Source: CAD feature listing. Evaluate the final solid. Frame: model axes, mm. Face numbers are marked on the shaded views. A direction names the side the tool comes from. Coordinates: 2 decimals unless noted, no trailing zeros. Loops run counter-clockwise (first coordinate to the right, second up) from the corner with the lowest first, then second, coordinate; pieces in that order, holes last. Notation, with made-up numbers: (47.25, 89) - (90.25, 89) arc R8 cw to (90.25, 102) - close; hole circle Ø1 at (70, 57.5). An arc over 180 degrees is marked (long way). Use one line per item in the form item = value. Start each with the question number.
from build123d import *

# Parameters (mm, degrees)
SKETCH1_W           = 36
SKETCH1_H           = 35
BOSS_EXTRUDE1_DEPTH = 11
SKETCH1_3_W         = 15
SKETCH1_3_H         = 35
BOSS_EXTRUDE2_DEPTH = 15.2
SKETCH2_W           = 31
SKETCH2_H           = 11.2
CUT_EXTRUDE1_DEPTH  = 1


with BuildPart() as part:
    # Sketch1 → Boss-Extrude1 (new body)
    with BuildSketch(Plane(origin=(0, 0, 0), x_dir=(1, 0, 0), z_dir=(0, 1, 0))):
        with Locations((-7.5, 0)):
            Rectangle(SKETCH1_W, SKETCH1_H)
    extrude(amount=BOSS_EXTRUDE1_DEPTH)

    # Sketch1<3> → Boss-Extrude2 (add)
    with BuildSketch(Plane(origin=(0, 0, 0), x_dir=(1, 0, 0), z_dir=(0, 1, 0))):
        with Locations((18, 0)):
            Rectangle(SKETCH1_3_W, SKETCH1_3_H)
    extrude(amount=BOSS_EXTRUDE2_DEPTH)

    # Sketch2 → Cut-Extrude1 (cut)
    with BuildSketch(Plane(origin=(25.5, 0, 0), x_dir=(0, 0, -1), z_dir=(1, 0, 0))):
        with Locations((0, 7.6)):
            Rectangle(SKETCH2_W, SKETCH2_H)
    extrude(amount=-CUT_EXTRUDE1_DEPTH, mode=Mode.SUBTRACT)


solid = part.part
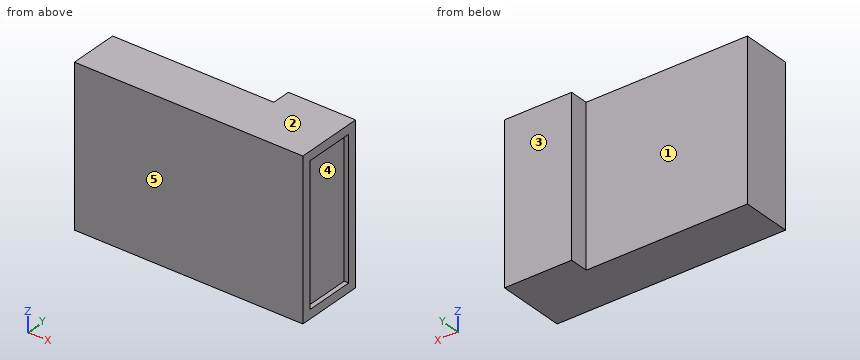
(1) Cut plane C-C, the plane x = -2. Output: boundary loops of the cut face in (y, z), plus the area to 3 significant figures.
(2) Mould query, pull axis Y, two halves, no side actions, for the marked faces 3, 4 and 5. Classes: +Y half, -Y half, draft (parallel to the pull), parting line (faces both ways), or undercut.
(3) Cut plane A-A, the plane y = 9.25. Output: boundary loops of the cut face in (x, z), plus the area to 3 significant figures.
(4) Cut plane D-D, the plane y = 14. Output: boundary loops of the cut face in (x, z).
(5) Access query for the marked faces 1 and 2. Directions: +Z, -Z, +X, -X, +Y, -Y. A direction counts if a zero-diameter tool reaches every point of the face in a straight line with its end or side. Return the directions, or none.
(6) Material intervals for line 1 (X direction, y = 11.5, z = -6); line 2 (Y direction, x = -14, z = 6); line 3 (X direction, y = 9.75, z = -13), sorted ascending.
(7) Contact query for flat-ended pins moving along their axis: pin 1 (6 mm diameter, centred on y = 5.5, z = 8.5, fed in from +X); pin 2 (10.5 mm diameter, centred on x = -4.5, z = 1.5, fed in from +Y). Output: stop coordinate, or through.
(8) Cut plane B-B, the plane z = 5. Output: boundary loops of the cut face in (x, y), plus the area to 3 significant figures.
Recorded:
q1.outline = (0, -17.5) - (11, -17.5) - (11, 17.5) - (0, 17.5) - close
q1.area = 385 mm²
q2.face_3 = +Y half
q2.face_4 = undercut
q2.face_5 = -Y half
q3.outline = (-25.5, -17.5) - (25.5, -17.5) - (25.5, -15.5) - (24.5, -15.5) - (24.5, 15.5) - (25.5, 15.5) - (25.5, 17.5) - (-25.5, 17.5) - close
q3.area = 1,750 mm²
q4.outline = (10.5, -17.5) - (25.5, -17.5) - (25.5, 17.5) - (10.5, 17.5) - close
q5.face_1 = +Z, -Z, -X, +Y
q5.face_2 = +Z, +X, -X, +Y, -Y
q6.line_1 = 10.5 to 24.5
q6.line_2 = 0 to 11
q6.line_3 = -25.5 to 24.5
q7.pin_1 = 24.5
q7.pin_2 = 11
q8.outline = (-25.5, 0) - (25.5, 0) - (25.5, 2) - (24.5, 2) - (24.5, 13.2) - (25.5, 13.2) - (25.5, 15.2) - (10.5, 15.2) - (10.5, 11) - (-25.5, 11) - close
q8.area = 613 mm²
